Work out the finished part from the listing and answer in its coordinate system (mm). Give positions to 0.01 mm unless a question says otherwise; leave off trailing zeros. Loops run counter-clockwise (first coordinate to the right, second up) from the corner with the lowest first, then second, coordinate; pieces in that order, holes last. Notation, with made-up numbers: M 40,62.5 L 87,62.5 A33 cw 87,98.5 Z; hole C 76.25,87.25 d7. An arc over 180 degrees is marked long. Write item = value, one per line. Start each with the question number.
1. Consider L1, parallel to X at y = -67, z = 38.25; L2, parallel to Y at x = -29, z = 40; L3, parallel to X at y = -9.5, z = 38. Determine where each line is inside the solid, lowest interval first. Write a range as [from, to].
2. Section B-B on x = -35.5 is taken. Determine the outline of the cut face in (y, z).
3. Flat-ended cylindrical pins translate along their axes: pin 1 Ø8 at (x, y) = (8, -55) entering from -Z; pin 2 Ø3 at (x, z) = (-12, 45.5) entering from +Y; pin 3 Ø6 at (y, z) = (-50.5, 32) entering from -X; pin 4 Ø5 at (x, z) = (-11, 38) entering from -Y. Find the tip coordinate at first contact, or state that the pin passes through.
4. Section D-D on y = -9.5 is taken. Determine the outline of the cut face in (x, z), plus the area to 3 significant figures.
5. Section A-A on z = 35 is taken. Determine the outline of the cut face in (x, y).
6. Section C-C on x = -14 is taken. Determine the outline of the cut face in (y, z).
7. The mould has two halves that part along X. Classify faces 1 (the face through (-14, -22.86, 39)), 2 (the face through (-36.92, -11.27, 32.88)), 3 (the face through (24.857, -11, 38)), 4 (the face through (7.083, -54.166, 38.902)): released by +X, released by -X, zero draft, split by the parting line, or undercut.
```python
from build123d import *

# Parameters (mm, degrees)
F0_W     = 76.2
F0_H     = 22.86
F0_R     = 6.477
F1_DEPTH = 22.86
F2_R     = 6.35
F3_DEPTH = 63.5


with BuildPart() as f1:
    # F0 (on Front) → F1 (new body)
    with BuildSketch(Plane.XZ):
        with Locations((-13.242823, 38.622339)):
            Rectangle(F0_W, F0_H)
        with Locations((-39.912823, 38.622339)):
            Circle(F0_R, mode=Mode.SUBTRACT)
    extrude(amount=F1_DEPTH)

    # F2 (on face) → F3 (join)
    with BuildSketch(Plane.XZ.offset(22.86)):
        with Locations((13.427177, 38.622339)):
            Circle(F2_R)
    extrude(amount=F3_DEPTH)


solid = f1.part
```
Verdict:
q1.L1 = [7.09, 19.77]
q1.L2 = [-22.86, 0]
q1.L3 = [-51.34, -46.36], [-33.47, 24.86]
q2.outline = M -22.86,27.19 L 0,27.19 L 0,33.88 L -22.86,33.88 Z; M -22.86,43.36 L 0,43.36 L 0,50.05 L -22.86,50.05 Z
q3.pin_1 = 32.43
q3.pin_2 = 0
q3.pin_3 = 8.21
q3.pin_4 = -22.86
q4.outline = M -51.34,27.19 L 24.86,27.19 L 24.86,50.05 L -51.34,50.05 Z; hole C -39.91,38.62 d12.95
q4.area = 1,610 mm2
q5.outline = M -51.34,-22.86 L -45.28,-22.86 L -45.28,0 L -51.34,0 Z; M -34.54,-22.86 L 8.21,-22.86 L 8.21,-86.36 L 18.64,-86.36 L 18.64,-22.86 L 24.86,-22.86 L 24.86,0 L -34.54,0 Z
q6.outline = M -22.86,27.19 L 0,27.19 L 0,50.05 L -22.86,50.05 Z
q7.face_1 = zero draft
q7.face_2 = undercut
q7.face_3 = released by +X
q7.face_4 = split by the parting line
